```python
from build123d import *

# Parameters (mm, degrees)
BOSS_EXTRUDE1_DEPTH             = 38.1
CUT_EXTRUDE1_DEPTH              = 100.190170884
CUT_EXTRUDE1_DEPTH_BACK         = 100.190170884
BOSS_EXTRUDE2_REACH             = 101.19
BOSS_EXTRUDE2_DIRECTION_2_REACH = 101.19
CUT_EXTRUDE2_DEPTH              = 100.190170884
CUT_EXTRUDE2_DEPTH_BACK         = 100.190170884
SKETCH5_W                       = 149.86
SKETCH5_H                       = 76.2
BOSS_EXTRUDE4_DEPTH             = 19.05
SKETCH6_R                       = 3.175
CUT_EXTRUDE3_DEPTH              = 188.543158451


with BuildPart() as part:
    # Sketch1 → Boss-Extrude1 (new body)
    with BuildSketch(Plane(origin=(44.224720049, 74.891650501, 130.282900288), x_dir=(1, 0, 0), z_dir=(0, 1, 0))):
        Polygon((-73.66, -50.8), (-73.66, -19.05), (-76.2, -19.05), (-76.2, 19.05), (-73.66, 19.05), (-73.66, 50.8), (73.66, 50.8), (73.66, 38.1), (76.2, 38.1), (76.2, -38.1), (73.66, -38.1), (73.66, -50.8), align=None)
    extrude(amount=BOSS_EXTRUDE1_DEPTH)

    # Sketch2 → Cut-Extrude1 (cut, two sides: drawn at the far end of the back side and taken through both)
    with BuildSketch(Plane(origin=(44.224720049, 74.891650501, 130.282900288), x_dir=(1, 0, 0), z_dir=(0, 0, 1)).offset(-CUT_EXTRUDE1_DEPTH_BACK)):
        Polygon((-76.2, 12.7), (-57.783825767, 21.287603079), (-55.084357434, 33.987603079), (-44.45, 38.1), (-76.2, 38.1), align=None)
        Polygon((32.670048754, 38.1), (76.2, 7.62), (76.2, 38.1), align=None)
    extrude(amount=CUT_EXTRUDE1_DEPTH + CUT_EXTRUDE1_DEPTH_BACK, mode=Mode.SUBTRACT)

    # Boss-Extrude2: up to this face of the body (flat: up to its plane)
    boss_extrude2_end = Plane(part.part.faces().sort_by_distance((41.857775963, 91.970339861, 181.082900288))[0])
    # Sketch3 → Boss-Extrude2 (add, up to the picked face)
    with BuildSketch(Plane(origin=(44.224720049, 74.891650501, 130.282900288), x_dir=(1, 0, 0), z_dir=(0, 0, 1)), mode=Mode.PRIVATE) as boss_extrude2_sk1:
        Polygon((-76.2, 0), (-76.2, -12.7), (-68.867651581, 0), align=None)
    boss_extrude2_tool1 = split(extrude(boss_extrude2_sk1.sketch, amount=BOSS_EXTRUDE2_REACH, mode=Mode.PRIVATE), bisect_by=boss_extrude2_end, keep=Keep.BOTH, mode=Mode.PRIVATE)
    # Sketch3 → Boss-Extrude2 (add, up to the picked face)
    with BuildSketch(Plane(origin=(44.224720049, 74.891650501, 130.282900288), x_dir=(1, 0, 0), z_dir=(0, 0, 1)), mode=Mode.PRIVATE) as boss_extrude2_sk2:
        Polygon((76.2, 0), (76.2, -12.7), (68.867651581, 0), align=None)
    boss_extrude2_tool2 = split(extrude(boss_extrude2_sk2.sketch, amount=BOSS_EXTRUDE2_REACH, mode=Mode.PRIVATE), bisect_by=boss_extrude2_end, keep=Keep.BOTH, mode=Mode.PRIVATE)
    add(boss_extrude2_tool1.solids().sort_by(Axis((-29.531164, 70.658317, 130.2829), (0, 0, 1)))[0])
    add(boss_extrude2_tool2.solids().sort_by(Axis((117.980604, 70.658317, 130.2829), (0, 0, 1)))[0])

    # Boss-Extrude2 direction 2: up to this face of the body (flat: up to its plane)
    boss_extrude2_direction_2_end = Plane(part.part.faces().sort_by_distance((41.857775963, 91.970339861, 79.482900288))[0])
    # Sketch3 → Boss-Extrude2 direction 2 (add, up to the picked face)
    with BuildSketch(Plane(origin=(44.224720049, 74.891650501, 130.282900288), x_dir=(1, 0, 0), z_dir=(0, 0, 1)), mode=Mode.PRIVATE) as boss_extrude2_direction_2_sk1:
        Polygon((-76.2, 0), (-76.2, -12.7), (-68.867651581, 0), align=None)
    boss_extrude2_direction_2_tool1 = split(extrude(boss_extrude2_direction_2_sk1.sketch, amount=-BOSS_EXTRUDE2_DIRECTION_2_REACH, mode=Mode.PRIVATE), bisect_by=boss_extrude2_direction_2_end, keep=Keep.BOTH, mode=Mode.PRIVATE)
    # Sketch3 → Boss-Extrude2 direction 2 (add, up to the picked face)
    with BuildSketch(Plane(origin=(44.224720049, 74.891650501, 130.282900288), x_dir=(1, 0, 0), z_dir=(0, 0, 1)), mode=Mode.PRIVATE) as boss_extrude2_direction_2_sk2:
        Polygon((76.2, 0), (76.2, -12.7), (68.867651581, 0), align=None)
    boss_extrude2_direction_2_tool2 = split(extrude(boss_extrude2_direction_2_sk2.sketch, amount=-BOSS_EXTRUDE2_DIRECTION_2_REACH, mode=Mode.PRIVATE), bisect_by=boss_extrude2_direction_2_end, keep=Keep.BOTH, mode=Mode.PRIVATE)
    add(boss_extrude2_direction_2_tool1.solids().sort_by(Axis((-29.531164, 70.658317, 130.2829), (0, 0, -1)))[0])
    add(boss_extrude2_direction_2_tool2.solids().sort_by(Axis((117.980604, 70.658317, 130.2829), (0, 0, -1)))[0])

    # Sketch4 → Cut-Extrude2 (cut, two sides: drawn at the far end of the back side and taken through both)
    with BuildSketch(Plane(origin=(44.224720049, 74.891650501, 130.282900288), x_dir=(0, 0, -1), z_dir=(1, 0, 0)).offset(-CUT_EXTRUDE2_DEPTH_BACK)):
        Polygon((-38.1, 38.1), (-50.8, 25.4), (-50.8, 38.1), align=None)
        Polygon((38.1, 38.1), (50.8, 25.4), (50.8, 38.1), align=None)
    extrude(amount=CUT_EXTRUDE2_DEPTH + CUT_EXTRUDE2_DEPTH_BACK, mode=Mode.SUBTRACT)

    # Sketch5 → Boss-Extrude4 (add)
    with BuildSketch(Plane.XZ.offset(-74.891650501)):
        with Locations((45.494720049, 130.282900288)):
            Rectangle(SKETCH5_W, SKETCH5_H)
    extrude(amount=BOSS_EXTRUDE4_DEPTH)

    # Sketch6 → Cut-Extrude3 (cut, through all)
    with BuildSketch(Plane(origin=(0, 0, 92.182900288), x_dir=(-1, 0, 0), z_dir=(0, 0, -1))):
        with Locations((-103.914720049, 61.216355026)):
            Circle(SKETCH6_R)
        with Locations((-45.494720049, 61.216355026)):
            Circle(SKETCH6_R)
        with Locations((12.925279951, 61.216355026)):
            Circle(SKETCH6_R)
    extrude(amount=-CUT_EXTRUDE3_DEPTH, mode=Mode.SUBTRACT)


solid = part.part
```
Here's how the part is built. I have some questions about the finished solid (model axes, mm). A direction names the side the tool comes from. Coordinates: 2 decimals unless noted, no trailing zeros. Order: outer loops, then holes, each group sorted by start corner. A loop starts at its lowest first (then second) coordinate and runs counter-clockwise, first axis right, second up.
Item 1: Thinking about a two-plate mould opening in X: for faces 4 (the face through (98.355, 97.965, 129.572)), 5 (the face through (-22.896, 91.825, 129.572)), 6 (the face through (44, 55.842, 131)), 7 (the face through (44, 66, 168.383)), which applies, pulls with the +X half, pulls with the -X half, needs draft (parallel to the pull), parting line crosses it, or undercut?
Response values:
face 4: pulls with the +X half
face 5: pulls with the -X half
face 6: needs draft
face 7: undercut
Item 2: If we section it at B-B, the plane z = 86: List the corners of the cut face in (x, y) for me.
Response values:
outline: (-31.98, 62.19) - (-24.64, 74.89) - (113.09, 74.89) - (120.42, 62.19) - (120.42, 74.89) - (117.88, 74.89) - (117.88, 84.29) - (85.72, 106.81) - (-11.3, 106.81) - (-13.56, 96.18) - (-29.44, 88.78) - (-29.44, 74.89) - (-31.98, 74.89) - close
Item 3: If we section it at A-A, the plane x = 28.5: List the corners of the cut face in (y, z) for me.
Response values:
outline: (55.84, 92.18) - (74.89, 92.18) - (74.89, 79.48) - (100.29, 79.48) - (112.99, 92.18) - (112.99, 168.38) - (100.29, 181.08) - (74.89, 181.08) - (74.89, 168.38) - (55.84, 168.38) - close
Item 4: If we section it at D-D, the plane y = 105: List the corners of the cut face in (x, z) for me.
Response values:
outline: (-11.68, 84.19) - (88.31, 84.19) - (88.31, 176.37) - (-11.68, 176.37) - close
Item 5: If we section it at C-C, the plane z = 131: List the corners of the cut face in (x, y) for me (3 decimals).
Response values:
outline: (-31.975, 62.192) - (-29.435, 66.591) - (-29.435, 55.842) - (120.425, 55.842) - (120.425, 82.512) - (76.895, 112.992) - (-0.225, 112.992) - (-10.86, 108.879) - (-13.559, 96.179) - (-31.975, 87.592) - close; hole circle Ø6.35 at (-12.925, 61.216); hole circle Ø6.35 at (45.495, 61.216); hole circle Ø6.35 at (103.915, 61.216)
Item 6: I need wall thicknesses on probe 1 along Y at (x, z) = (48, 101.5); probe 2 along Y at (x, z) = (-14.5, 142.5); probe 3 along Z at (x, y) = (54, 71). Which ranges of each line are inside material? Lowest first, please.
Response values:
probe 1: y = 55.84 to 59.27, 63.17 to 112.99
probe 2: y = 55.84 to 58.46, 63.97 to 95.74
probe 3: z = 92.18 to 168.38
Item 7: I'm going to push flat-ended pins straight in: pin 1 Ø6 at (x, y) = (-5.5, 103) entering from -Z; pin 2 Ø4 at (x, y) = (65.5, 65.5) entering from -Z; pin 3 Ø5 at (x, y) = (76, 105) entering from +Z; pin 4 Ø4 at (x, y) = (45.49, 61.22) entering from +Z. Where does each tip first touch, or does it pass through?
Response values:
pin 1: stops at z = 79.48
pin 2: stops at z = 92.18
pin 3: stops at z = 178.87
pin 4: passes through
Item 8: Which directions (+Z, -Z, +X, -X, +Y, -Y) give clear straight access to the entire face, cutting with the end or side of a thin tool? Please do faces 1 (the face through (-29.435, 82, 165)), 2 (the face through (-29.435, 82, 96)), 3 (the face through (44, 66, 92.183)).
Response values:
face 1: +Z, -X, +Y
face 2: -Z, -X, +Y
face 3: -Z, -Y
